Can you work these out from the model? Positions are in its coordinate system, mm. Give positions to 0.01 mm unless a question says otherwise; leave off trailing zeros. Order: outer loops, then holes, each group sorted by start corner. A loop starts at its lowest first (then second) coordinate and runs counter-clockwise, first axis right, second up. Notation, with made-up numbers: (11.5, -35.5) - (37.5, -35.5) arc R16 ccw to (37.5, -11.5) - close; hole circle Ø4 at (49.25, 28). An arc over 180 degrees is marked (long way). Answer as CSV lines item,"result".
```python
from build123d import *

# Parameters (mm, degrees)
SKETCH1_W           = 6.35
SKETCH1_H           = 1.778
BOSS_EXTRUDE1_DEPTH = 1.5875
CUT_EXTRUDE1_REACH  = 38.738
SKETCH2_W           = 3.155094666
SKETCH2_H           = 2.647438771
FILLET1_R           = 1.778
FILLET2_R           = 0.762
FILLET3_R           = 0.762
SKETCH3_R           = 0.6096
CUT_EXTRUDE2_DEPTH  = 1.5875


with BuildPart() as part:
    # Sketch1 → Boss-Extrude1 (new body)
    # profile 1 of 3: a face of its own
    with BuildSketch(Plane.XY):
        with BuildLine():
            ThreePointArc((29.21, 13.97), (26.792166479, 19.807166479), (20.955, 22.225))
            Line((20.955, 22.225), (-20.955, 22.225))
            ThreePointArc((-20.955, 22.225), (-26.792166479, 19.807166479), (-29.21, 13.97))
            Line((-29.21, 13.97), (-29.21, -13.97))
            ThreePointArc((-29.21, -13.97), (-26.792166479, -19.807166479), (-20.955, -22.225))
            Line((-20.955, -22.225), (20.955, -22.225))
            ThreePointArc((20.955, -22.225), (26.792166479, -19.807166479), (29.21, -13.97))
            Line((29.21, -13.97), (29.21, 13.97))
        make_face()
        with BuildLine():
            Line((-9.632094666, -18.923), (-20.955, -18.923))
            ThreePointArc((-20.955, -18.923), (-24.457299887, -17.472299887), (-25.908, -13.97))
            Line((-25.908, -13.97), (-25.908, -1.27))
            Line((-25.908, -1.27), (-25.908, -0.381))
            Line((-25.908, -0.381), (-25.908, 0))
            Line((-25.908, 0), (-25.908, 1.397))
            Line((-25.908, 1.397), (-25.908, 13.97))
            ThreePointArc((-25.908, 13.97), (-24.457299887, 17.472299887), (-20.955, 18.923))
            Line((-20.955, 18.923), (20.955, 18.923))
            ThreePointArc((20.955, 18.923), (24.457299887, 17.472299887), (25.908, 13.97))
            Line((25.908, 13.97), (25.908, 1.397))
            Line((25.908, 1.397), (25.908, -0.381))
            Line((25.908, -0.381), (25.908, -13.97))
            ThreePointArc((25.908, -13.97), (24.457299887, -17.472299887), (20.955, -18.923))
            Line((20.955, -18.923), (9.632094666, -18.923))
            Line((9.632094666, -18.923), (2.416367182, -12.868285729))
            ThreePointArc((2.416367182, -12.868285729), (0, -19.5072), (-2.416367182, -12.868285729))
            Line((-2.416367182, -12.868285729), (-9.632094666, -18.923))
        make_face(mode=Mode.SUBTRACT)
    # profile 2 of 3: a face of its own
    with BuildSketch(Plane.XY):
        with Locations((22.733, 0.508)):
            Rectangle(SKETCH1_W, SKETCH1_H)
    # profile 3 of 3: a face of its own
    with BuildSketch(Plane.XY):
        Polygon((-25.908, 0), (-25.908, -0.381), (-19.558, -0.381), (-19.558, 1.397), (-25.908, 1.397), align=None)
    extrude(amount=BOSS_EXTRUDE1_DEPTH)

    # Sketch2 → Cut-Extrude1 (cut, up to next)
    with BuildSketch(Plane.XY.offset(1.5875), mode=Mode.PRIVATE) as cut_extrude1_sk1:
        with Locations((-8.054547333, -17.599280615)):
            Rectangle(SKETCH2_W, SKETCH2_H)
    cut_extrude1_tool1 = extrude(cut_extrude1_sk1.sketch, amount=-CUT_EXTRUDE1_REACH, mode=Mode.PRIVATE) & part.part
    # Sketch2 → Cut-Extrude1 (cut, up to next)
    with BuildSketch(Plane.XY.offset(1.5875), mode=Mode.PRIVATE) as cut_extrude1_sk2:
        with Locations((8.054547333, -17.599280615)):
            Rectangle(SKETCH2_W, SKETCH2_H)
    cut_extrude1_tool2 = extrude(cut_extrude1_sk2.sketch, amount=-CUT_EXTRUDE1_REACH, mode=Mode.PRIVATE) & part.part
    # Sketch2 → Cut-Extrude1 (cut, up to next)
    with BuildSketch(Plane.XY.offset(1.5875), mode=Mode.PRIVATE) as cut_extrude1_sk3:
        with BuildLine():
            Line((-20.955, 18.923), (20.955, 18.923))
            ThreePointArc((20.955, 18.923), (21.595374802, 18.881428419), (22.225, 18.757411514))
            Line((22.225, 18.757411514), (22.225, 22.225))
            Line((22.225, 22.225), (-22.225, 22.225))
            Line((-22.225, 22.225), (-22.225, 18.757411514))
            ThreePointArc((-22.225, 18.757411514), (-21.595374802, 18.881428419), (-20.955, 18.923))
        make_face()
    cut_extrude1_tool3 = extrude(cut_extrude1_sk3.sketch, amount=-CUT_EXTRUDE1_REACH, mode=Mode.PRIVATE) & part.part
    add(cut_extrude1_tool1.solids().sort_by_distance((-8.054547, -17.599281, 1.5875))[0], mode=Mode.SUBTRACT)
    add(cut_extrude1_tool2.solids().sort_by_distance((8.054547, -17.599281, 1.5875))[0], mode=Mode.SUBTRACT)
    add(cut_extrude1_tool3.solids().sort_by_distance((0, 20.572388, 1.5875))[0], mode=Mode.SUBTRACT)

    # Fillet1
    fillet1_edges = [part.edges().sort_by_distance(p)[0] for p in [
        (-6.477, -18.923, 0.79375),
        (-6.477, -16.275561229, 0.79375),
        (6.477, -18.923, 0.79375),
        (6.477, -16.275561229, 0.79375),
    ]]
    fillet(fillet1_edges, radius=FILLET1_R)

    # Fillet2
    fillet2_edges = [part.edges().sort_by_distance(p)[0] for p in [
        (-22.225, 22.126722687, 0.79375),
        (-22.225, 18.757411514, 0.79375),
        (22.225, 18.757411514, 0.79375),
        (22.225, 22.126722687, 0.79375),
    ]]
    fillet(fillet2_edges, radius=FILLET2_R)

    # Fillet3
    fillet3_edges = [part.edges().sort_by_distance(p)[0] for p in [
        (25.908, -0.381, 0.79375),
        (25.908, 1.397, 0.79375),
        (-25.908, 1.397, 0.79375),
        (-25.908, -0.381, 0.79375),
    ]]
    fillet(fillet3_edges, radius=FILLET3_R)

    # Sketch3 → Cut-Extrude2 (cut)
    with BuildSketch(Plane.XY.offset(1.5875)):
        with Locations((-26.289, 17.78)):
            Circle(SKETCH3_R)
        with Locations((-25.781, -18.034)):
            Circle(SKETCH3_R)
        with Locations((26.289, 17.78)):
            Circle(SKETCH3_R)
        with Locations((25.781, -18.034)):
            Circle(SKETCH3_R)
    extrude(amount=-CUT_EXTRUDE2_DEPTH, mode=Mode.SUBTRACT)


solid = part.part
```
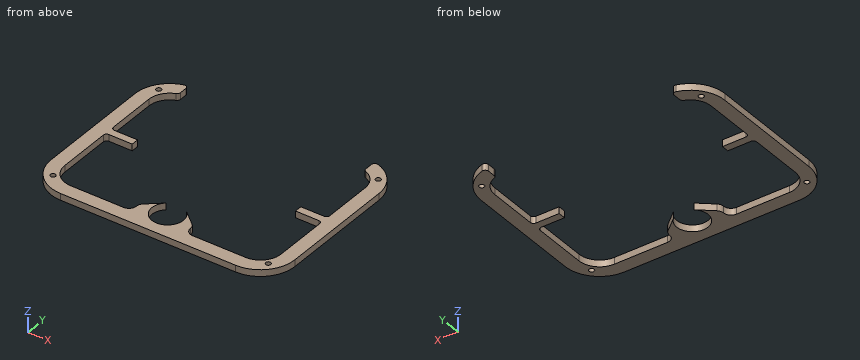
1) I'm going to push a flat-ended pin straight in: P1, Ø0.8, axis at x = 21.5, z = 0.5, coming from the -Y side. Where does the tip first touch, or does it pass through?
Answer block:
P1,"y = -22.22"
2) I want a section at A-A on y = -8. Write out the boundary of the cut face in (x, z).
Answer block:
outline,"(-29.21, 0) - (-25.91, 0) - (-25.91, 1.59) - (-29.21, 1.59) - close; (25.91, 0) - (29.21, 0) - (29.21, 1.59) - (25.91, 1.59) - close"
3) I want a section at D-D on z = 1.2. Count the separate pieces of the cut face and the enclosed holes in it, plus the area to 3 significant figures.
Answer block:
separate pieces,"1"
enclosed holes,"4"
area,"494 mm2"
4) I want a section at C-C on x = -14. Write out the boundary of the cut face in (y, z) (1 decimal).
Answer block:
outline,"(-22.2, 0) - (-18.9, 0) - (-18.9, 1.6) - (-22.2, 1.6) - close"
5) I want a section at B-B on y = 17.78. Write out the boundary of the cut face in (x, z), plus the area to 3 significant figures.
Answer block:
outline,"(-28.28, 0) - (-26.9, 0) - (-26.9, 1.59) - (-28.28, 1.59) - close; (-25.68, 0) - (-24.12, 0) - (-24.12, 1.59) - (-25.68, 1.59) - close; (24.12, 0) - (25.68, 0) - (25.68, 1.59) - (24.12, 1.59) - close; (26.9, 0) - (28.28, 0) - (28.28, 1.59) - (26.9, 1.59) - close"
area,"9.33 mm2"
6) I need wall thicknesses on line 1 along X through (y, z) = (5, 0.3); line 2 along Y through (x, z) = (25, 1.3); line 3 along X through (y, z) = (18, 1.1). Which ranges of each line are inside material? Lowest first, please. Write a range as [from, to].
Answer block:
line 1,"[-29.21, -25.91], [25.91, 29.21]"
line 2,"[-21.17, -16.83], [-0.38, 1.4], [16.83, 21.17]"
line 3,"[-28.16, -26.86], [-25.72, -23.83], [23.83, 25.72], [26.86, 28.16]"
